CAD build for the part. Positions are in the model's coordinates, mm. A direction names the side the tool comes from. Coordinates: 2 decimals unless noted, no trailing zeros. Loops run counter-clockwise (first coordinate to the right, second up) from the corner with the lowest first, then second, coordinate; pieces in that order, holes last. Notation, with made-up numbers: (12, 75.25) - (34, 75.25) arc R15 cw to (34, 102.25) - close; hole circle Ø10 at (-13.5, 15.5). An arc over 180 degrees is marked (long way). Put each result on its own line as item: value.
```python
from build123d import *

# Parameters (mm, degrees)
SKETCH1_W                                    = 101.6
SKETCH1_H                                    = 19.812
BOSS_EXTRUDE1_DEPTH                          = 3.81
CSK_FOR_M6_COUNTERSUNK_FLAT_HEAD_SCR_2_COUNT = 2
CSK_FOR_M6_COUNTERSUNK_FLAT_HEAD_SCR_2_PITCH = 59.69
SKETCH5_W                                    = 101.6
SKETCH5_H                                    = 19.812
SKETCH5_R                                    = 6.3
BOSS_EXTRUDE2_DEPTH                          = 3.81
SKETCH6_R                                    = 3.175
CUT_EXTRUDE1_DEPTH                           = 6.35
CUT_EXTRUDE2_DEPTH                           = 7.35
CUT_EXTRUDE2_DEPTH_BACK                      = 14.462


with BuildPart() as part:
    # Sketch1 → Boss-Extrude1 (new body)
    with BuildSketch(Plane(origin=(0, 0, 0), x_dir=(1, 0, 0), z_dir=(0, 1, 0))):
        Rectangle(SKETCH1_W, SKETCH1_H)
    extrude(amount=BOSS_EXTRUDE1_DEPTH)

    # Sketch4 → CSK for M6 Countersunk Flat Head Screw1 (revolve, cut)
    with BuildSketch(Plane(origin=(-29.845, 3.81, 1.651), x_dir=(0, 0, 1), z_dir=(1, 0, 0))):
        Polygon((0, 0), (0, 3.81), (3.5, 3.81), (3.5, 3.054), (6.3, 0.254), (6.3, 0), align=None)
    csk_for_m6_countersunk_flat_head_screw1 = revolve(axis=Axis((-29.845, 10.16, 1.651), (0, -1, 0)), mode=Mode.SUBTRACT)

    # CSK for M6 Countersunk Flat Head Scr 2: CSK for M6 Countersunk Flat Head Screw1 ×2
    with Locations(*[(i * CSK_FOR_M6_COUNTERSUNK_FLAT_HEAD_SCR_2_PITCH, 0, 0) for i in range(1, CSK_FOR_M6_COUNTERSUNK_FLAT_HEAD_SCR_2_COUNT)]):
        add(csk_for_m6_countersunk_flat_head_screw1, mode=Mode.SUBTRACT)

    # Sketch5 → Boss-Extrude2 (add)
    with BuildSketch(Plane(origin=(0, 3.81, 0), x_dir=(1, 0, 0), z_dir=(0, 1, 0))):
        Rectangle(SKETCH5_W, SKETCH5_H)
        with Locations((-29.845, -1.651)):
            Circle(SKETCH5_R, mode=Mode.SUBTRACT)
        with Locations((29.845, -1.651)):
            Circle(SKETCH5_R, mode=Mode.SUBTRACT)
    extrude(amount=BOSS_EXTRUDE2_DEPTH)

    # Sketch6 → Cut-Extrude1 (cut)
    with BuildSketch(Plane(origin=(0, 0, -9.906), x_dir=(-1, 0, 0), z_dir=(0, 0, -1))):
        with Locations((0, 7.874)):
            Circle(SKETCH6_R)
    extrude(amount=-CUT_EXTRUDE1_DEPTH, mode=Mode.SUBTRACT)

    # Sketch7 → Cut-Extrude2 (cut, two sides)
    with BuildSketch(Plane(origin=(0, 0, -3.556), x_dir=(-1, 0, 0), z_dir=(0, 0, -1))) as cut_extrude2_sk:
        with BuildLine():
            ThreePointArc((-2.36766458, 7.62), (0, 5.49275), (2.36766458, 7.62))
            Line((2.36766458, 7.62), (-2.36766458, 7.62))
        make_face()
        with BuildLine():
            Line((-2.36766458, 7.62), (2.36766458, 7.62))
            ThreePointArc((2.36766458, 7.62), (2.377851219, 7.746818473), (2.38125, 7.874))
            ThreePointArc((2.38125, 7.874), (-0.127181527, 10.251851219), (-2.36766458, 7.62))
        make_face()
    extrude(amount=CUT_EXTRUDE2_DEPTH, mode=Mode.SUBTRACT)
    extrude(cut_extrude2_sk.sketch, amount=-CUT_EXTRUDE2_DEPTH_BACK, mode=Mode.SUBTRACT)


solid = part.part
```
Q1. Tool access for faces 1 (the flat face through (-27, 7.62, -5)), 2 (the flat face through (0, 5, -3.556)): list every direction of +Z, -Z, +X, -X, +Y, -Y with a clear straight run to the whole face (end or side of a thin tool).
Determined:
face 1: +Z, -Z, +X, -X, +Y
face 2: -Z, +Y
Q2. Slice it at C-C, the plane z = 3.5. State how many separate pieces and enclosed holes the cut face has, then the cut area to 3 significant figures.
Determined:
separate pieces: 3
enclosed holes: 0
area: 609 mm2
Q3. Pin check, flat tips, straight feed: pin 1 Ø7.5 at (x, z) = (29.845, 1.651) entering from -Y; pin 2 Ø11 at (x, z) = (29.845, 1.651) entering from +Y; pin 3 Ø10 at (x, z) = (-29.845, 1.651) entering from +Y. Stop position of each tip, or through.
Determined:
pin 1: y = 0
pin 2: y = 2.76
pin 3: y = 2.26
Q4. Mould opens along X. For faces 3 (the flat face through (-50.8, 4, 0)), 4 (the cylindrical face through (0.1, 4.7, -6.8)), 5 (the flat face through (50.8, 4, 0)), 6 (the flat face through (-1, 4, 9.906)) say: +X half, -X half, draft (parallel to the pull), parting line (faces both ways), or undercut.
Determined:
face 3: -X half
face 4: undercut
face 5: +X half
face 6: draft
Q5. Wall check: L1, parallel to X at y = 3.75, z = 6.25; L2, parallel to X at y = 2.75, z = 6.5; L3, parallel to X at y = 6.75, z = 4. Give the ranges that are in metal, low to high. Write a range as from..to.
Determined:
L1: -50.8..-34.15, -25.54..25.54, 34.15..50.8
L2: -50.8..-32.43, -27.26..27.26, 32.43..50.8
L3: -50.8..-35.69, -24..-2.1, 2.1..24, 35.69..50.8
Q6. Slice it at A-A, the plane z = -7.5. Give the cut face in (x, y) (3 decimals).
Determined:
outline: (-50.8, 0) - (50.8, 0) - (50.8, 7.62) - (3.165, 7.62) arc R3.175 cw to (-3.165, 7.62) - (-50.8, 7.62) - close
Q7. Slice it at B-B, the plane y = 2. Give the cut face in (x, z) (3 decimals).
Determined:
outline: (-50.8, -9.906) - (50.8, -9.906) - (50.8, 9.906) - (-50.8, 9.906) - close; hole circle Ø9.488 at (-29.845, 1.651); hole circle Ø9.488 at (29.845, 1.651)
